from build123d import *

# Parameters (mm, degrees)
BOSS_EXTRUDE1_DEPTH = 13
BOSS_EXTRUDE2_DEPTH = 3
CUT_EXTRUDE1_START  = -3
SKETCH2_W           = 16
SKETCH2_H           = 5.5
CUT_EXTRUDE1_DEPTH  = 3


with BuildPart() as part:
    # Sketch1 → Boss-Extrude1 (new body)
    with BuildSketch(Plane.XY):
        with BuildLine():
            Line((-10.5, 40.1497198), (-10.5, 48.597279697))
            Line((-10.5, 48.597279697), (10.5, 48.597279697))
            Line((10.5, 48.597279697), (10.5, 40.1497198))
            ThreePointArc((10.5, 40.1497198), (11.251983463, 39.945498722), (12, 39.727194716))
            Line((12, 39.727194716), (12, 50.097279697))
            Line((12, 50.097279697), (-12, 50.097279697))
            Line((-12, 50.097279697), (-12, 39.727194716))
            ThreePointArc((-12, 39.727194716), (-11.251983463, 39.945498722), (-10.5, 40.1497198))
        make_face()
        with BuildLine():
            ThreePointArc((12, 39.727194716), (11.251983463, 39.945498722), (10.5, 40.1497198))
            Line((10.5, 40.1497198), (10.5, 38.597279697))
            ThreePointArc((10.5, 38.597279697), (11.252148087, 38.384751705), (12, 38.157568057))
            Line((12, 38.157568057), (12, 39.727194716))
        make_face()
        with BuildLine():
            Line((-12, 38.157568057), (-12, 39.727194716))
            ThreePointArc((-12, 39.727194716), (-24.741160037, -33.318538383), (41.5, 0))
            ThreePointArc((41.5, 0), (33.318538383, 24.741160037), (12, 39.727194716))
            Line((12, 39.727194716), (12, 38.157568057))
            ThreePointArc((12, 38.157568057), (32.249030993, 23.664319132), (40, 0))
            ThreePointArc((40, 0), (-23.664319132, -32.249030993), (-12, 38.157568057))
        make_face()
        with BuildLine():
            Line((-10.5, 38.597279697), (-10.5, 40.1497198))
            ThreePointArc((-10.5, 40.1497198), (-11.251983463, 39.945498722), (-12, 39.727194716))
            Line((-12, 39.727194716), (-12, 38.157568057))
            ThreePointArc((-12, 38.157568057), (-11.252148087, 38.384751705), (-10.5, 38.597279697))
        make_face()
    extrude(amount=-BOSS_EXTRUDE1_DEPTH)

    # Sketch1_3 → Boss-Extrude2 (add)
    with BuildSketch(Plane.XY):
        with BuildLine():
            Line((-12, 37.097279697), (-12, 38.157568057))
            ThreePointArc((-12, 38.157568057), (-23.664319132, -32.249030993), (40, 0))
            ThreePointArc((40, 0), (32.249030993, 23.664319132), (12, 38.157568057))
            Line((12, 38.157568057), (12, 37.097279697))
            Line((12, 37.097279697), (-12, 37.097279697))
        make_face()
        with BuildLine():
            Line((10.5, 38.597279697), (-10.5, 38.597279697))
            ThreePointArc((-10.5, 38.597279697), (-11.252148087, 38.384751705), (-12, 38.157568057))
            Line((-12, 38.157568057), (-12, 37.097279697))
            Line((-12, 37.097279697), (12, 37.097279697))
            Line((12, 37.097279697), (12, 38.157568057))
            ThreePointArc((12, 38.157568057), (11.252148087, 38.384751705), (10.5, 38.597279697))
        make_face()
        with BuildLine():
            ThreePointArc((10.5, 38.597279697), (0, 40), (-10.5, 38.597279697))
            Line((-10.5, 38.597279697), (10.5, 38.597279697))
        make_face()
        with BuildLine():
            ThreePointArc((10.5, 40.1497198), (0, 41.5), (-10.5, 40.1497198))
            Line((-10.5, 40.1497198), (-10.5, 38.597279697))
            ThreePointArc((-10.5, 38.597279697), (0, 40), (10.5, 38.597279697))
            Line((10.5, 38.597279697), (10.5, 40.1497198))
        make_face()
        with BuildLine():
            Line((10.5, 48.597279697), (-10.5, 48.597279697))
            Line((-10.5, 48.597279697), (-10.5, 40.1497198))
            ThreePointArc((-10.5, 40.1497198), (0, 41.5), (10.5, 40.1497198))
            Line((10.5, 40.1497198), (10.5, 48.597279697))
        make_face()
    extrude(amount=-BOSS_EXTRUDE2_DEPTH)

    # Sketch2 → Cut-Extrude1 (cut)
    with BuildSketch(Plane.XY.offset(CUT_EXTRUDE1_START)):
        with Locations((0, 43.347279697)):
            Rectangle(SKETCH2_W, SKETCH2_H)
    extrude(amount=CUT_EXTRUDE1_DEPTH, mode=Mode.SUBTRACT)


solid = part.part
Verification items for the finished model (mm, model axes). A direction names the side the tool comes from. Coordinates: 2 decimals unless noted, no trailing zeros. Order: outer loops, then holes, each group sorted by start corner. A loop starts at its lowest first (then second) coordinate and runs counter-clockwise, first axis right, second up. Notation, with made-up numbers: M 63,-4 L 83,-4 A20 cw 83,29 Z; hole C -2,34.5 d2. An arc over 180 degrees is marked long. One line per item, written item: value. Start each with the question number.
Item 1: Sectioned sample at C-C (y = 2.5). Enter the section's corners in (x, z), then the cut area to 3 significant figures.
Item 2: Scan lines: probe 1 along Y at (x, z) = (0, -10.25); probe 2 along X at (y, z) = (42, -4.25); probe 3 along X at (y, z) = (0, -11). Record each from-to range of solid material in increasing order.
Item 3: Sectioned sample at B-B (z = -5.75). Enter the section's corners in (x, y).
Item 4: Mould release check, pull along Y, two halves, no side actions. Record for faces 1 (the flat face through (0, 50.097, -6)), 2 (the flat face through (-25, 32, -13)), 3 (the flat face through (0, 46.097, -2)): released by +Y, released by -Y, zero draft, split by the parting line, or undercut.
Item 5: Sectioned sample at D-D (x = 27). Enter the section's corners in (y, z).
Item 6: Gauge pin test, flat ends, axial feed: pin 1 (2 mm diameter, centred on y = 22, z = -6.5, fed in from +X); pin 2 (2.5 mm diameter, centred on y = 43.5, z = -1, fed in from -X); pin 3 (0.9 mm diameter, centred on x = 2.5, z = -2, fed in from -Y). Record the tip position at first contact, or that the pin passes through.
Item 7: Access from +Z, -Z, +X, -X, +Y, -Y to the whole of each face (thin tool, end or side, straight path). Record for faces 4 (the flat face through (12, 45, -6)), 5 (the flat face through (-12, 45, -6)), 6 (the flat face through (-10.5, 44, -8)), 7 (the flat face through (8, 43, -2)).
Item 8: Sectioned sample at A-A (x = 0). Enter the section's corners in (y, z).
Conclusion:
1. outline: M -41.42,-13 L -39.92,-13 L -39.92,-3 L 39.92,-3 L 39.92,-13 L 41.42,-13 L 41.42,0 L -41.42,0 Z
1. area: 279 mm^2
2. probe 1: y = -41.5 to -40, 48.6 to 50.1
2. probe 2: x = -12 to -10.5, 10.5 to 12
2. probe 3: x = -41.5 to -40, 40 to 41.5
3. outline: M -12,39.73 A41.5 ccw long 12,39.73 L 12,50.1 L -12,50.1 Z; hole M -10.5,38.6 A40 ccw long 10.5,38.6 L 10.5,48.6 L -10.5,48.6 Z
4. face 1: released by +Y
4. face 2: zero draft
4. face 3: undercut
5. outline: M -31.52,-13 L -29.51,-13 L -29.51,-3 L 29.51,-3 L 29.51,-13 L 31.52,-13 L 31.52,0 L -31.52,0 Z
6. pin 1: stops at x = 35.79
6. pin 2: stops at x = -12
6. pin 3: stops at y = -41.45
7. face 4: +Z, -Z, +X, +Y
7. face 5: +Z, -Z, -X, +Y
7. face 6: -Z
7. face 7: +Z, -Z
8. outline: M -41.5,-13 L -40,-13 L -40,-3 L 40.6,-3 L 40.6,0 L -41.5,0 Z; M 46.1,-3 L 48.6,-3 L 48.6,-13 L 50.1,-13 L 50.1,0 L 46.1,0 Z
